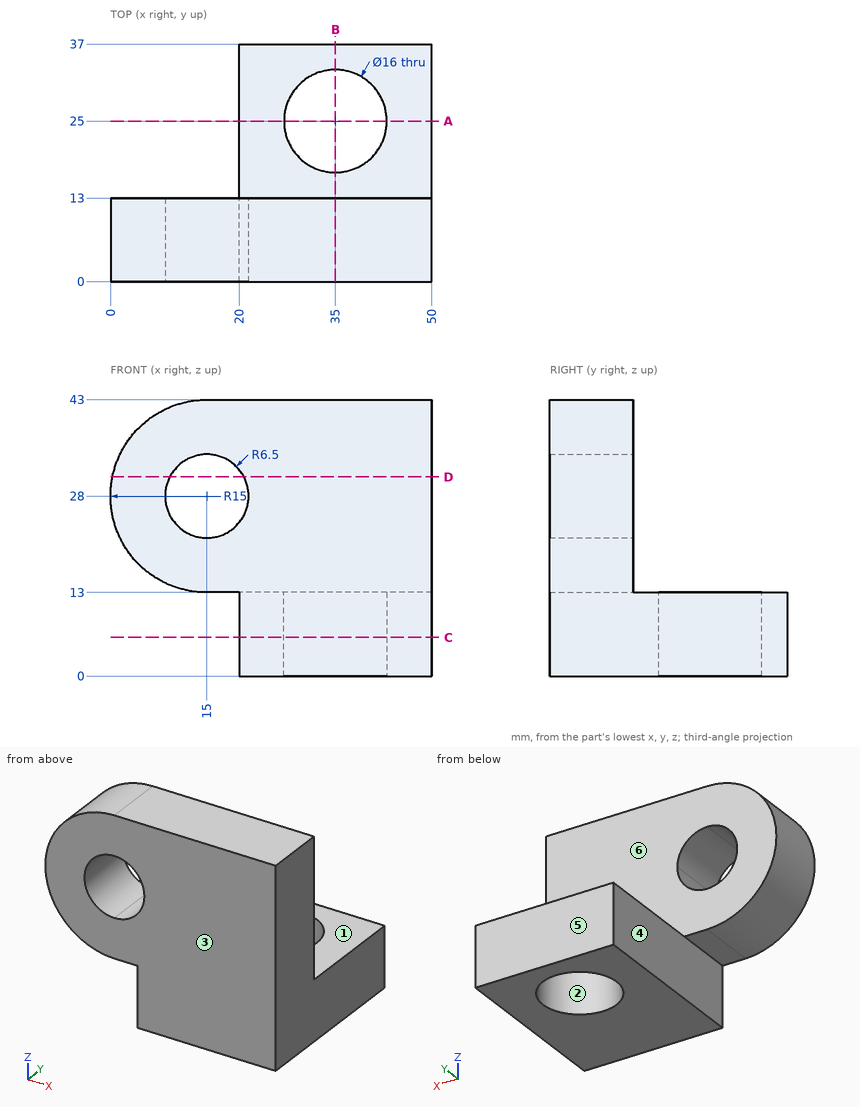
Design review of the part shown in the three views and the two pictorial views. Dimensions are in mm from the part's minimum x, y and z. A direction names the side the tool comes from. Round coordinates to 2 decimals unless told otherwise and drop trailing zeros. Order: outer loops, then holes, each group sorted by start corner. A loop starts at its lowest first (then second) coordinate and runs counter-clockwise, first axis right, second up. Notation, with made-up numbers: (63, -2.5) - (77, -2.5) arc R18 cw to (77, 17.5) - close; hole circle Ø10 at (61.5, 86). An arc over 180 degrees is marked (long way). One line per question, with ' | ' between items.
Item 1: Take a section at B-B, the plane x = 35. Write out the cut boundary in (y, z), then the cut area to 3 significant figures.
Checks:
outline: (0, 0) - (17, 0) - (17, 13) - (13, 13) - (13, 43) - (0, 43) - close; (33, 0) - (37, 0) - (37, 13) - (33, 13) - close | area: 663 mm²
Item 2: Wall thickness on line 1 (Y direction, x = 35, z = 4); line 2 (Z direction, x = 25, y = 26.5); line 3 (X direction, y = 29, z = 2.5): over which ranges is each line inside the solid? List them lowest first. Write a range as [from, to].
Checks:
line 1: [0, 17], [33, 37] | line 2: [0, 13] | line 3: [20, 28.07], [41.93, 50]
Item 3: Take a section at D-D, the plane z = 31. Write out the cut boundary in (x, y), then the cut area to 3 significant figures.
Checks:
outline: (0.3, 0) - (9.23, 0) - (9.23, 13) - (0.3, 13) - close; (20.77, 0) - (50, 0) - (50, 13) - (20.77, 13) - close | area: 496 mm²
Item 4: For P1, Ø1, axis at x = 36, z = 27, coming from the +Y side; P2, Ø8, axis at x = 37, y = 20, coming from the +Z side; P3, Ø10.5, axis at y = 23, z = 5, coming from the -X side, all flat-tipped, find the tip position at first contact; note any pin that passes through.
Checks:
P1: y = 13 | P2: z = 13 | P3: x = 20
Item 5: Take a section at A-A, the plane y = 25. Write out the cut boundary in (x, z), then the cut area to 3 significant figures.
Checks:
outline: (20, 0) - (27, 0) - (27, 13) - (20, 13) - close; (43, 0) - (50, 0) - (50, 13) - (43, 13) - close | area: 182 mm²
Item 6: Machinability: for the marked faces 4, 5 and 6, which of the approach directions +Z, -Z, +X, -X, +Y, -Y give a long, thin tool a straight path to every point of the face, cutting with its end or side? Answer none if there is none.
Checks:
face 4: -Z, -X, +Y, -Y | face 5: +Z, -Z, +X, -X, +Y | face 6: +Z, +X, -X, +Y
Item 7: Take a section at C-C, the plane z = 6. Write out the cut boundary in (x, y).
Checks:
outline: (20, 0) - (50, 0) - (50, 37) - (20, 37) - close; hole circle Ø16 at (35, 25)
Item 8: Draft analysis for pull direction Y (two halves, no side actions). For the marked faces 1, 2 and 3, state which applies: +Y half, -Y half, draft (parallel to the pull), parting line (faces both ways), or undercut.
Checks:
face 1: draft | face 2: undercut | face 3: -Y half
